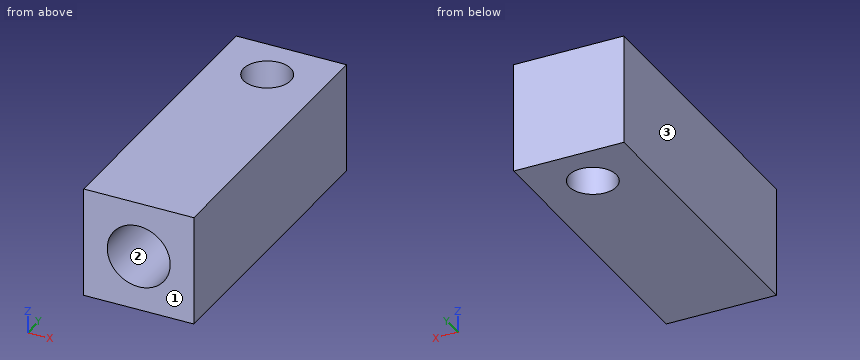
```python
from build123d import *

# Parameters (mm, degrees)
SKETCH1_W                       = 7
SKETCH1_H                       = 7
SKETCH1_R                       = 2
BOSS_EXTRUDE1_DEPTH             = 13
BOSS_EXTRUDE2_REACH             = 5.5
SKETCH2_W                       = 7
SKETCH2_H                       = 6
SKETCH2_R                       = 1.5
BOSS_EXTRUDE2_DIRECTION_2_REACH = 5.5


with BuildPart() as part:
    # Sketch1 → Boss-Extrude1 (new body)
    with BuildSketch(Plane(origin=(0, 0, 0), x_dir=(1, 0, 0), z_dir=(0, 1, 0))):
        Rectangle(SKETCH1_W, SKETCH1_H)
        Circle(SKETCH1_R, mode=Mode.SUBTRACT)
    extrude(amount=BOSS_EXTRUDE1_DEPTH)

    # Boss-Extrude2: up to this face of the body (flat: up to its plane)
    boss_extrude2_end = Plane(part.part.faces().sort_by_distance((0, 6.5, 3.5))[0])
    # Sketch2 → Boss-Extrude2 (add, up to the picked face)
    with BuildSketch(Plane.XY, mode=Mode.PRIVATE) as boss_extrude2_sk1:
        with Locations((0, 16)):
            Rectangle(SKETCH2_W, SKETCH2_H)
        with Locations((0, 16)):
            Circle(SKETCH2_R, mode=Mode.SUBTRACT)
    boss_extrude2_tool1 = split(extrude(boss_extrude2_sk1.sketch, amount=BOSS_EXTRUDE2_REACH, mode=Mode.PRIVATE), bisect_by=boss_extrude2_end, keep=Keep.BOTH, mode=Mode.PRIVATE)
    add(boss_extrude2_tool1.solids().sort_by_distance((0, 18.907805, 0))[0])

    # Boss-Extrude2 direction 2: up to this face of the body (flat: up to its plane)
    boss_extrude2_direction_2_end = Plane(part.part.faces().sort_by_distance((0, 6.5, -3.5))[0])
    # Sketch2 → Boss-Extrude2 direction 2 (add, up to the picked face)
    with BuildSketch(Plane.XY, mode=Mode.PRIVATE) as boss_extrude2_direction_2_sk1:
        with Locations((0, 16)):
            Rectangle(SKETCH2_W, SKETCH2_H)
        with Locations((0, 16)):
            Circle(SKETCH2_R, mode=Mode.SUBTRACT)
    boss_extrude2_direction_2_tool1 = split(extrude(boss_extrude2_direction_2_sk1.sketch, amount=-BOSS_EXTRUDE2_DIRECTION_2_REACH, mode=Mode.PRIVATE), bisect_by=boss_extrude2_direction_2_end, keep=Keep.BOTH, mode=Mode.PRIVATE)
    add(boss_extrude2_direction_2_tool1.solids().sort_by_distance((0, 18.907805, 0))[0])


solid = part.part
```
Geometry check sheet. Reference: the model listing, model coordinates, mm. Face numbers are marked on the shaded views. Give positions to 0.01 mm unless a question says otherwise; leave off trailing zeros. Write each loop counter-clockwise with the first axis right and the second up, starting at its lowest first coordinate (ties: lowest second). Pieces come first, ordered by that corner, then holes. Notation, with made-up numbers: (-20.75, 57.25) -> (18.25, 57.25) arc R14 ccw to (18.25, 65.25) -> close; hole circle Ø11 at (-15, 71.25). An arc over 180 degrees is marked (long way). Use one line per item in the form item = value.
Item 1: Sectioned sample at B-B on y = 16. Enter the section's corners in (x, z).
Results list:
outline = (-3.5, -3.5) -> (-1.5, -3.5) -> (-1.5, 3.5) -> (-3.5, 3.5) -> close; (1.5, -3.5) -> (3.5, -3.5) -> (3.5, 3.5) -> (1.5, 3.5) -> close
Item 2: Mould release check, pull along X, two halves, no side actions. Record for the marked faces 1, 2 and 3: released by +X, released by -X, zero draft, split by the parting line, or undercut.
Results list:
face_1 = zero draft
face_2 = undercut
face_3 = released by -X
Item 3: Sectioned sample at A-A on z = 0. Enter the section's corners in (x, y), plus the area to 3 significant figures.
Results list:
outline = (-3.5, 0) -> (-2, 0) -> (-2, 13) -> (2, 13) -> (2, 0) -> (3.5, 0) -> (3.5, 19) -> (-3.5, 19) -> close; hole circle Ø3 at (0, 16)
area = 73.9 mm2
Item 4: Sectioned sample at D-D on y = 6.25. Enter the section's corners in (x, z).
Results list:
outline = (-3.5, -3.5) -> (3.5, -3.5) -> (3.5, 3.5) -> (-3.5, 3.5) -> close; hole circle Ø4 at (0, 0)
Item 5: Scan lines: line 1 (X direction, y = 9.25, z = 0); line 2 (X direction, y = 16, z = 0.25). Record each from-to range of solid material in increasing order.
Results list:
line_1 = -3.5 to -2, 2 to 3.5
line_2 = -3.5 to -1.5, 1.5 to 3.5
Item 6: Sectioned sample at C-C on x = 0. Enter the section's corners in (y, z).
Results list:
outline = (0, -3.5) -> (14.5, -3.5) -> (14.5, 3.5) -> (0, 3.5) -> (0, 2) -> (13, 2) -> (13, -2) -> (0, -2) -> close; (17.5, -3.5) -> (19, -3.5) -> (19, 3.5) -> (17.5, 3.5) -> close
Item 7: Depth check by flat-ended pin: pin 1 Ø3.5 at (x, y) = (0, 16) entering from +Z. Enter the tip coordinate at first touch or a pass-through.
Results list:
pin_1 = 3.5
